Read the model definition and answer for the solid it produces. Units are mm, in the model's axes. Face numbers are marked on the shaded views. A direction names the side the tool comes from. Give positions to 0.01 mm unless a question says otherwise; leave off trailing zeros. Write each loop counter-clockwise with the first axis right and the second up, starting at its lowest first coordinate (ties: lowest second). Pieces come first, ordered by that corner, then holes. Notation, with made-up numbers: (-1.5, -7.75) - (34.5, -7.75) arc R20 cw to (34.5, -0.75) - close; hole circle Ø6 at (-15.5, -20). An arc over 180 degrees is marked (long way). Answer as a JSON object with one key per item and string values. Group by question number.
```python
from build123d import *

# Parameters (mm, degrees)
SKETCH2_W           = 121.92
SKETCH2_H           = 71.12
BOSS_EXTRUDE1_DEPTH = 12.7
SKETCH3_R           = 31.75
BOSS_EXTRUDE2_DEPTH = 11.43


with BuildPart() as part:
    # Sketch2 → Boss-Extrude1 (new body)
    with BuildSketch(Plane.XY):
        Rectangle(SKETCH2_W, SKETCH2_H)
    extrude(amount=-BOSS_EXTRUDE1_DEPTH)

    # Sketch3 → Boss-Extrude2 (add)
    with BuildSketch(Plane.XY):
        with BuildLine():
            Line((-13.67831861, 35.56), (13.67831861, 35.56))
            ThreePointArc((13.67831861, 35.56), (38.1, 0), (13.67831861, -35.56))
            Line((13.67831861, -35.56), (-13.67831861, -35.56))
            ThreePointArc((-13.67831861, -35.56), (-38.1, 0), (-13.67831861, 35.56))
        make_face()
        Circle(SKETCH3_R, mode=Mode.SUBTRACT)
    extrude(amount=BOSS_EXTRUDE2_DEPTH)


solid = part.part
```
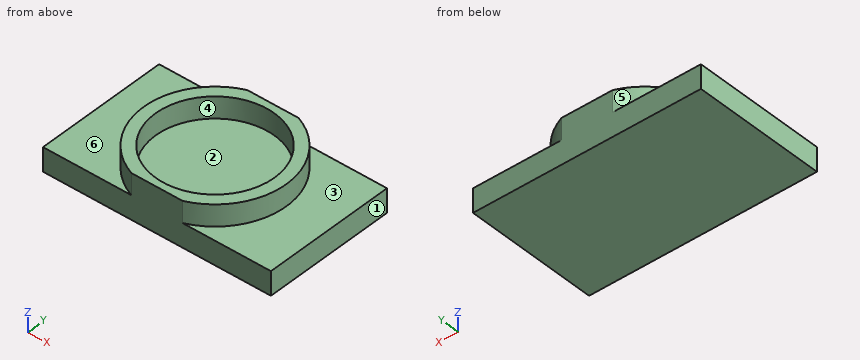
1) Flat-ended cylindrical pins translate along their axes: pin 1 Ø12 at (y, z) = (16, 8.5) entering from +X; pin 2 Ø12 at (x, y) = (1.5, -20) entering from +Z; pin 3 Ø12 at (y, z) = (24.5, 7.5) entering from +X. Find the tip coordinate at first contact, or state that the pin passes through.
2) Find section D-D, the plane y = 29. Write down the section's boundary in (x, z), and give its area (3 significant figures).
3) Which of the six approach directions +Z, -Z, +X, -X, +Y, -Y give full straight-line access (tool end or side, diameter ignored) to the marked faces 1, 2 and 3?
4) Find the intervals of material crossed by line 1 (Y direction, x = 0, z = 3.5); line 2 (Z direction, x = -4, y = 12.5); line 3 (X direction, y = -24.5, z = 6.5), in increasing order. Write a range as [from, to].
5) Find section A-A, the plane z = 9.5. Write down the section's boundary in (x, y).
6) Find section C-C, the plane y = 0. Write down the section's boundary in (x, z).
7) Find section B-B, the plane x = 0. Write down the section's boundary in (y, z), and give its area (3 significant figures).
8) For a pull along X with two mould halves and no side action, classify the marked faces 4, 5 and 6 as released by +X, released by -X, zero draft, split by the parting line, or undercut.
Values follow:
{
 "1": {"pin 1": "stops at x = 36.76", "pin 2": "stops at z = 0", "pin 3": "stops at x = 33.31"},
 "2": {"outline": "(-60.96, -12.7) - (60.96, -12.7) - (60.96, 0) - (24.71, 0) - (24.71, 11.43) - (12.93, 11.43) - (12.93, 0) - (-12.93, 0) - (-12.93, 11.43) - (-24.71, 11.43) - (-24.71, 0) - (-60.96, 0) - close", "area": "1,820 mm2"},
 "3": {"face 1": "+Z, -Z, +X, +Y, -Y", "face 2": "+Z", "face 3": "+Z, +X"},
 "4": {"line 1": "y = [-35.56, -31.75], [31.75, 35.56]", "line 2": "z = [-12.7, 0]", "line 3": "x = [-29.18, -20.19], [20.19, 29.18]"},
 "5": {"outline": "(-13.68, -35.56) - (13.68, -35.56) arc R38.1 ccw to (13.68, 35.56) - (-13.68, 35.56) arc R38.1 ccw to start; hole circle Ø63.5 at (0, 0)"},
 "6": {"outline": "(-60.96, -12.7) - (60.96, -12.7) - (60.96, 0) - (38.1, 0) - (38.1, 11.43) - (31.75, 11.43) - (31.75, 0) - (-31.75, 0) - (-31.75, 11.43) - (-38.1, 11.43) - (-38.1, 0) - (-60.96, 0) - close"},
 "7": {"outline": "(-35.56, -12.7) - (35.56, -12.7) - (35.56, 11.43) - (31.75, 11.43) - (31.75, 0) - (-31.75, 0) - (-31.75, 11.43) - (-35.56, 11.43) - close", "area": "990 mm2"},
 "8": {"face 4": "undercut", "face 5": "released by -X", "face 6": "zero draft"}
}
